from build123d import *

# Parameters (mm, degrees)
SKETCH3_W           = 2.9591
SKETCH3_H           = 6.35
BOSS_EXTRUDE1_DEPTH = 1.47955


with BuildPart() as part:
    # Sketch3 → Boss-Extrude1 (new body, symmetric)
    with BuildSketch(Plane.XY):
        Polygon((-12.7, 6.35), (12.7, 6.35), (12.7, 4.7625), (18.415, 4.7625), (18.415, -4.7625), (12.7, -4.7625), (12.7, -6.35), (-12.7, -6.35), (-12.7, -4.7625), (-18.415, -4.7625), (-18.415, 4.7625), (-12.7, 4.7625), align=None)
        with Locations((-5.41655, 0)):
            Rectangle(SKETCH3_W, SKETCH3_H, mode=Mode.SUBTRACT)
        with Locations((5.41655, 0)):
            Rectangle(SKETCH3_W, SKETCH3_H, mode=Mode.SUBTRACT)
    extrude(amount=BOSS_EXTRUDE1_DEPTH, both=True)


solid = part.part
Input: part model. Units: mm. Frame: model coordinates. A direction names the side the tool comes from. Round coordinates to 2 decimals unless told otherwise and drop trailing zeros. Loops run counter-clockwise (first coordinate to the right, second up) from the corner with the lowest first, then second, coordinate; pieces in that order, holes last. Notation, with made-up numbers: (-36.5, -20) -> (-9.5, -20) arc R15 cw to (-9.5, 6) -> close; hole circle Ø7 at (-20, 43.5). An arc over 180 degrees is marked (long way). Answer as a JSON object with one key per item and string values. Group by question number.
1) Draft query along Y for faces 6 (the flat face through (-16, 4.762, 0)), 7 (the flat face through (16, -4.762, 0)), 8 (the flat face through (-5, -3.175, 0)), 9 (the flat face through (-18.415, 0, 0)). Return one class per face: +Y half, -Y half, draft (parallel to the pull), parting line (faces both ways), or undercut.
2) Reachability of faces 1 (the flat face through (12.7, 6, 0)), 2 (the flat face through (-12.7, 6, 0)), 3 (the flat face through (-16, -4.762, 0)), 4 (the flat face through (12.7, -6, 0)), 5 (the flat face through (6.896, 0, 0)) from +Z, -Z, +X, -X, +Y, -Y: full face, straight path, thin tool, end or side. Return the list, or none.
3) Ray query, L1, parallel to X at y = 2.75, z = 0.75 (3 decimals); L2, parallel to Y at x = 5, z = 1.15 (3 decimals); L3, parallel to X at y = 5, z = -0.1. Return the intervals inside material, ascending.
4) Pin query (flat end, axial travel): pin 1 (1.3 mm diameter, centred on y = -5.5, z = 0.5, fed in from +X); pin 2 (1.3 mm diameter, centred on y = -5.5, z = 0, fed in from -X); pin 3 (0.9 mm diameter, centred on x = 14.5, z = 0.5, fed in from -Y). Return the tip coordinate at first contact, or that it passes through.
5) Section query B-B on x = -6.5. Output: boundary loops of the cut face in (y, z) (3 decimals), plus the area to 3 significant figures.
6) Section query A-A on y = 1.25. Output: boundary loops of the cut face in (x, z) (3 decimals), plus the area to 3 significant figures.
7) Section query C-C on z = 1. State how many separate pieces and enclosed holes the cut face has, plus the area to 3 significant figures.
8) Section query D-D on y = -5.25. Output: boundary loops of the cut face in (x, z).
Reply:
{
 "1": {"face 6": "+Y half", "face 7": "-Y half", "face 8": "undercut", "face 9": "draft"},
 "2": {"face 1": "+Z, -Z, +X, +Y", "face 2": "+Z, -Z, -X, +Y", "face 3": "+Z, -Z, -X, -Y", "face 4": "+Z, -Z, +X, -Y", "face 5": "+Z, -Z"},
 "3": {"L1": "x = -18.415 to -6.896, -3.937 to 3.937, 6.896 to 18.415", "L2": "y = -6.35 to -3.175, 3.175 to 6.35", "L3": "x = -12.7 to 12.7"},
 "4": {"pin 1": "stops at x = 12.7", "pin 2": "stops at x = -12.7", "pin 3": "stops at y = -4.76"},
 "5": {"outline": "(-6.35, -1.48) -> (-3.175, -1.48) -> (-3.175, 1.48) -> (-6.35, 1.48) -> close; (3.175, -1.48) -> (6.35, -1.48) -> (6.35, 1.48) -> (3.175, 1.48) -> close", "area": "18.8 mm2"},
 "6": {"outline": "(-18.415, -1.48) -> (-6.896, -1.48) -> (-6.896, 1.48) -> (-18.415, 1.48) -> close; (-3.937, -1.48) -> (3.937, -1.48) -> (3.937, 1.48) -> (-3.937, 1.48) -> close; (6.896, -1.48) -> (18.415, -1.48) -> (18.415, 1.48) -> (6.896, 1.48) -> close", "area": "91.5 mm2"},
 "7": {"separate pieces": "1", "enclosed holes": "2", "area": "394 mm2"},
 "8": {"outline": "(-12.7, -1.48) -> (12.7, -1.48) -> (12.7, 1.48) -> (-12.7, 1.48) -> close"}
}
